```python
from build123d import *

# Parameters (mm, degrees)
SKETCH2_R                 = 10.033
BOSS_EXTRUDE1_DEPTH       = 12.7
M3X0_5_TAPPED_HOLE1_D     = 2.5
M3X0_5_TAPPED_HOLE1_DEPTH = 10.16
M3X0_5_TAPPED_HOLE1_TIP   = 0.751075774


with BuildPart() as part:
    # Sketch1 → Revolve2 (revolve)
    with BuildSketch(Plane.XY):
        with BuildLine():
            Line((0, 0), (0, 133.068754945))
            ThreePointArc((0, 133.068754945), (0.686399651, 132.801828719), (1.012133813, 132.14130518))
            Line((1.012133813, 132.14130518), (12.573, 0))
            Line((12.573, 0), (0, 0))
        make_face()
    revolve(axis=Axis((0, 0, 0), (0, 1, 0)))

    # Sketch2 → Boss-Extrude1 (add)
    with BuildSketch(Plane.XZ):
        Circle(SKETCH2_R)
    extrude(amount=BOSS_EXTRUDE1_DEPTH)

    # M3x0.5 Tapped Hole1
    with Locations(Plane.XZ.offset(12.7)):
        with Locations((0, 0)):
            Hole(M3X0_5_TAPPED_HOLE1_D / 2, depth=M3X0_5_TAPPED_HOLE1_DEPTH)
            with Locations((0, 0, -(M3X0_5_TAPPED_HOLE1_DEPTH + M3X0_5_TAPPED_HOLE1_TIP / 2))):  # 118° drill point
                Cone(0, M3X0_5_TAPPED_HOLE1_D / 2, M3X0_5_TAPPED_HOLE1_TIP, mode=Mode.SUBTRACT)


solid = part.part
```
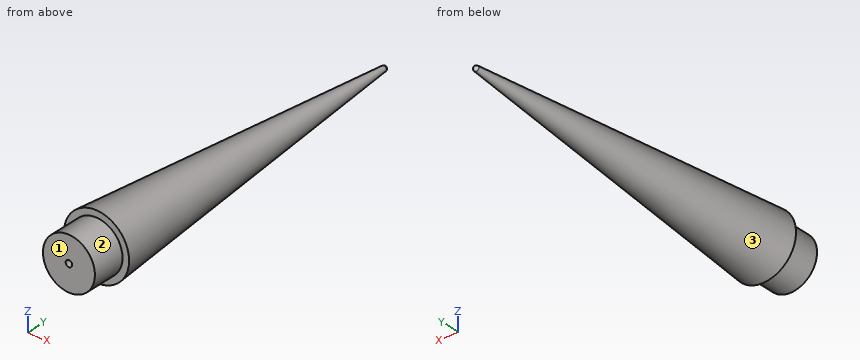
Design review of the part built by this model. Coordinates are the model's own, in mm. Face numbers are marked on the shaded views. Coordinates: 2 decimals unless noted, no trailing zeros. Write each loop counter-clockwise with the first axis right and the second up, starting at its lowest first coordinate (ties: lowest second). Pieces come first, ordered by that corner, then holes.
1) Insertion check: pin 1 (2 mm diameter, centred on y = 74.5, z = 6, fed in from -X); pin 2 (1.5 mm diameter, centred on y = 2, z = 5, fed in from -X); pin 3 (1.5 mm diameter, centred on y = 45.5, z = 7.5, fed in from -X). Each pin has a flat end and moves straight along its axis. Give the tip position at first contact, or say it passes through.
2) Add section B-B (y = 105.5). Write out the cut boundary in (x, z).
3) To check wall thickness, follow L1, parallel to Z at x = 0, y = -8.5; L2, parallel to X at y = 77.5, z = -1.75; L3, parallel to Z at x = -5.5, y = -6. State the ranges of each line that lie inside material, in increasing order.
4) Add section A-A (y = 37). Write out the cut boundary in (x, z).
5) Mouldability with a two-part tool opening along Y and no side actions: class the marked faces 1, 2 and 3 as +Y half, -Y half, draft (parallel to the pull), parting line (faces both ways), or undercut.
Check result:
1. pin 1: stops at x = -3.42
1. pin 2: stops at x = -11.66
1. pin 3: stops at x = -5.32
2. outline: circle Ø6.69 at (0, 0)
3. L1: z = -10.03 to -1.25, 1.25 to 10.03
3. L2: x = -5.52 to 5.52
3. L3: z = -8.39 to 8.39
4. outline: circle Ø18.67 at (0, 0)
5. face 1: -Y half
5. face 2: draft
5. face 3: +Y half
